Design review of the part built by this model. Coordinates are the model's own, in mm. A direction names the side the tool comes from. Coordinates: 2 decimals unless noted, no trailing zeros. Loops run counter-clockwise (first coordinate to the right, second up) from the corner with the lowest first, then second, coordinate; pieces in that order, holes last. Notation, with made-up numbers: M 8.25,6 L 34.25,6 A20 cw 34.25,45 Z; hole C -35,72 d5. An arc over 180 degrees is marked long. One line per item, written item: value.
```python
from build123d import *

# Parameters (mm, degrees)
F0_W     = 12
F0_H     = 11.57143
F1_DEPTH = 30
F2_R     = 1.7
F3_DEPTH = 30
F4_W     = 1
F4_H     = 10
F5_DEPTH = 6


with BuildPart() as f1:
    # F0 (on Top) → F1 (new body)
    with BuildSketch(Plane.XY):
        Rectangle(F0_W, F0_H)
    extrude(amount=F1_DEPTH)

    # F2 (on face) → F3 (cut)
    with BuildSketch(Plane.XY.offset(30)):
        Circle(F2_R)
    extrude(amount=-F3_DEPTH, mode=Mode.SUBTRACT)

    # F4 (on face) → F5 (cut)
    with BuildSketch(Plane.XZ.offset(5.785715)):
        with Locations((0, 15.774963)):
            Rectangle(F4_W, F4_H)
    extrude(amount=-F5_DEPTH, mode=Mode.SUBTRACT)


solid = f1.part
```
(1) To check wall thickness, follow line 1 along Y through (x, z) = (0, 23.75); line 2 along X through (y, z) = (-3.75, 18); line 3 along Z through (x, y) = (-0.25, -4.5). State the ranges of each line that lie inside material, in increasing order. Write a range as [from, to].
Reply:
line 1: y = [-5.79, -1.7], [1.7, 5.79]
line 2: x = [-6, -0.5], [0.5, 6]
line 3: z = [0, 10.77], [20.77, 30]
(2) Mouldability with a two-part tool opening along Z and no side actions: class faces 3 (the cylindrical face through (0.914, 1.433, 15.21)), 4 (the flat face through (1.25, 1.37, 0)), 5 (the flat face through (0.5, -4, 16)) as released by +Z, released by -Z, zero draft, split by the parting line, or undercut.
Reply:
face 3: zero draft
face 4: released by -Z
face 5: undercut
(3) We need section C-C on z = 21.25. State the section outline as (x, y) points.
Reply:
outline: M -6,-5.79 L 6,-5.79 L 6,5.79 L -6,5.79 Z; hole C 0,0 d3.4
(4) We need section B-B on y = 0. State the section outline as (x, z) points.
Reply:
outline: M -6,0 L -1.7,0 L -1.7,30 L -6,30 Z; M 1.7,0 L 6,0 L 6,30 L 1.7,30 Z
(5) We need section A-A on x = 0. State the section outline as (y, z) points, then the cut area to 3 significant figures.
Reply:
outline: M -5.79,0 L -1.7,0 L -1.7,10.77 L -5.79,10.77 Z; M -5.79,20.77 L -1.7,20.77 L -1.7,30 L -5.79,30 Z; M 1.7,0 L 5.79,0 L 5.79,30 L 1.7,30 Z
area: 204 mm2
(6) We need section D-D on y = -4.75. State the section outline as (x, z) points.
Reply:
outline: M -6,0 L 6,0 L 6,30 L -6,30 Z; hole M -0.5,10.77 L 0.5,10.77 L 0.5,20.77 L -0.5,20.77 Z
(7) Tool access review of faces 1 (the flat face through (-0.5, -4, 16)), 2 (the flat face through (6, 0, 15)): name each direction out of +Z, -Z, +X, -X, +Y, -Y from which nothing blocks a thin tool from reaching the whole face with its end or side.
Reply:
face 1: -Y
face 2: +Z, -Z, +X, +Y, -Y
